Here's how the part is built. I have some questions about the finished solid (model axes, mm). Round coordinates to 2 decimals unless told otherwise and drop trailing zeros. Loops run counter-clockwise (first coordinate to the right, second up) from the corner with the lowest first, then second, coordinate; pieces in that order, holes last. Notation, with made-up numbers: (1, 70.5) - (8, 70.5) arc R26 ccw to (8, 107.5) - close; hole circle Ø3 at (13, 36). An arc over 180 degrees is marked (long way). Answer as a JSON object with one key per item and string values. Group by question number.
1) If we mould it in two halves opening along X, with no side actions, what happens to faces 1 (the face through (8.82, 0.74, -1.09)), 2 (the face through (-10.875, 1, -1)), 3 (the face through (9.48, 0.74, 5.94))? For each: pulls with the +X half, pulls with the -X half, needs draft (parallel to the pull), parting line crosses it, or undercut.
2) Will these pins go through, and if not, where does the flat tip stop? P1, Ø4, axis at x = 1.5, z = 1, coming from the +Y side; P2, Ø8, axis at x = 3, z = -4.5, coming from the -Y side.
3) I want a section at A-A, the plane y = 1.15. Please give me the cut outline in (x, z) (3 decimals), then the cut area to 3 significant figures.
4) If I drill on line 1 along X through (y, z) = (1.2, -1.25) (3 decimals); line 2 along X through (y, z) = (0.2, -1.5) (3 decimals); line 3 along Y through (x, z) = (-3, 3.25), over which ranges is the centre line in solid material (lowest first)? Write a range as [from, to].
from build123d import *

# Parameters (mm, degrees)
ESQUISSE1_R             = 0.4
BOSS_EXTRU_1_DEPTH      = 1.5
ESQUISSE2_W             = 13
ESQUISSE2_H             = 14.75
ENL_V_MAT_EXTRU_1_DEPTH = 0.01


with BuildPart() as part:
    # Esquisse1 → Boss.-Extru.1 (new body)
    with BuildSketch(Plane(origin=(0, 0, 0), x_dir=(1, 0, 0), z_dir=(0, 1, 0))):
        Polygon((-10.875, 7.375), (10.875, 7.375), (10.875, -4.546572875), (8.046572875, -7.375), (-8.046572875, -7.375), (-10.875, -4.546572875), align=None)
        with Locations(Location((-9.175, 1.275, 0), (0, 0, 270))):
            Circle(ESQUISSE1_R, mode=Mode.SUBTRACT)
        with Locations(Location((-9.175, 3.975, 0), (0, 0, 270))):
            Circle(ESQUISSE1_R, mode=Mode.SUBTRACT)
        with Locations(Location((9.175, 1.275, 0), (0, 0, 270))):
            Circle(ESQUISSE1_R, mode=Mode.SUBTRACT)
        with Locations(Location((9.175, 3.975, 0), (0, 0, 270))):
            Circle(ESQUISSE1_R, mode=Mode.SUBTRACT)
    extrude(amount=BOSS_EXTRU_1_DEPTH)

    # Esquisse2 → Enlèv. mat.-Extru.1 (cut)
    with BuildSketch(Plane(origin=(0, 1.5, 0), x_dir=(1, 0, 0), z_dir=(0, 1, 0))):
        Rectangle(ESQUISSE2_W, ESQUISSE2_H)
    extrude(amount=-ENL_V_MAT_EXTRU_1_DEPTH, mode=Mode.SUBTRACT)


solid = part.part
Outcome:
{
 "1": {"face 1": "undercut", "face 2": "pulls with the -X half", "face 3": "pulls with the +X half"},
 "2": {"P1": "y = 1.49", "P2": "y = 0"},
 "3": {"outline": "(-10.875, -7.375) - (10.875, -7.375) - (10.875, 4.547) - (8.047, 7.375) - (-8.047, 7.375) - (-10.875, 4.547) - close; hole circle Ø0.8 at (-9.175, -3.975); hole circle Ø0.8 at (-9.175, -1.275); hole circle Ø0.8 at (9.175, -3.975); hole circle Ø0.8 at (9.175, -1.275)", "area": "311 mm^2"},
 "4": {"line 1": "[-10.875, -9.574], [-8.776, 8.776], [9.574, 10.875]", "line 2": "[-10.875, -9.506], [-8.844, 8.844], [9.506, 10.875]", "line 3": "[0, 1.49]"}
}
